from build123d import *

# Parameters (mm, degrees)
SKETCH_1_R           = 2.5
SKETCH_1_R_2         = 8
EXTRUDE_1_DEPTH      = 2
SKETCH_2_R           = 34
CUT_EXTRUDE_1_DEPTH  = 0.5
SKETCH_3_R           = 2
CUT_EXTRUDE_2_DEPTH  = 28.5
SKETCH_5_R           = 2.1
CUT_EXTRUDE_3_DEPTH  = 10
SKETCH_4_R           = 2.6
CUT_EXTRUDE_4_DEPTH  = 10
SKETCH_7_W           = 125
SKETCH_7_H           = 125
SKETCH_7_W_2         = 80
SKETCH_7_H_2         = 80
EXTRUDE_2_DEPTH      = 2
SKETCH_8_R           = 2.760887892
EXTRUDE_3_DEPTH      = 2
SKETCH_9_R           = 2.6
CUT_EXTRUDE_5_DEPTH  = 2
CUT_EXTRUDE_7_DEPTH  = 2
EXTRUDE_START        = -2
SKETCH_11_W          = 250
SKETCH_11_H          = 250
SKETCH_11_R          = 2.1
SKETCH_11_R_2        = 8
EXTRUDE_4_DEPTH      = 2
SKETCH_13_R          = 2.6
CUT_EXTRUDE_9_DEPTH  = 51
SKETCH_16_R          = 34
CUT_EXTRUDE_11_DEPTH = 1
SKETCH_18_W          = 250
SKETCH_18_H          = 250
SKETCH_18_W_2        = 90
SKETCH_18_H_2        = 90
CUT_EXTRUDE_12_DEPTH = 10
SKETCH_20_R          = 2.6
CUT_EXTRUDE_14_DEPTH = 10
SKETCH_21_R          = 8.1
CUT_EXTRUDE_15_DEPTH = 10
SKETCH_24_R          = 34.1
CUT_EXTRUDE_17_DEPTH = 1
EXTRUDE_START_2      = 1
SKETCH_25_R          = 34.1
SKETCH_25_R_2        = 2.1
SKETCH_25_R_3        = 8.1
EXTRUDE_5_DEPTH      = 1
CUT_EXTRUDE_20_DEPTH = 10
SKETCH_31_W          = 90
SKETCH_31_H          = 90
SKETCH_31_R          = 2.1
SKETCH_31_R_2        = 8.1
SKETCH_31_R_3        = 2.6
EXTRUDE_6_DEPTH      = 4
EXTRUDE_START_3      = -4
EXTRUDE_7_DEPTH      = 4
CUT_EXTRUDE_21_DEPTH = 10


with BuildPart() as part:
    # 草图1 → 凸台-拉伸1 (new body)
    with BuildSketch(Plane.XY):
        Polygon((-33, 40), (-40, 40), (-40, 33), (-40, -33), (-40, -40), (40, -40), (40, 40), (33, 40), align=None)
        with Locations((-33, -33)):
            Circle(SKETCH_1_R, mode=Mode.SUBTRACT)
        with Locations((33, -30.5)):
            Circle(SKETCH_1_R, mode=Mode.SUBTRACT)
        Circle(SKETCH_1_R_2, mode=Mode.SUBTRACT)
        with Locations((-33, 33)):
            Circle(SKETCH_1_R, mode=Mode.SUBTRACT)
        with Locations((33, 33)):
            Circle(SKETCH_1_R, mode=Mode.SUBTRACT)
    extrude(amount=EXTRUDE_1_DEPTH)

    # 草图2 → 切除-拉伸1 (cut)
    with BuildSketch(Plane.XY.offset(2)):
        Circle(SKETCH_2_R)
    extrude(amount=-CUT_EXTRUDE_1_DEPTH, mode=Mode.SUBTRACT)

    # 草图3 → 切除-拉伸2 (cut)
    with BuildSketch(Plane.XY.offset(1.5)):
        with Locations((0, 30)):
            Circle(SKETCH_3_R)
        with Locations((25.980762114, -15)):
            Circle(SKETCH_3_R)
        with Locations((-25.980762114, -15)):
            Circle(SKETCH_3_R)
    extrude(amount=-CUT_EXTRUDE_2_DEPTH, mode=Mode.SUBTRACT)

    # 草图5 → 切除-拉伸3 (cut)
    with BuildSketch(Plane.XY.offset(1.5)):
        with Locations((25.980762114, -15)):
            Circle(SKETCH_5_R)
        with Locations((0, 30)):
            Circle(SKETCH_5_R)
        with Locations((-25.980762114, -15)):
            Circle(SKETCH_5_R)
    extrude(amount=-CUT_EXTRUDE_3_DEPTH, mode=Mode.SUBTRACT)

    # 草图4 → 切除-拉伸4 (cut)
    with BuildSketch(Plane.XY.offset(2)):
        with Locations((-33, 33)):
            Circle(SKETCH_4_R)
        with Locations((33, 33)):
            Circle(SKETCH_4_R)
        with Locations((33, -30.5)):
            Circle(SKETCH_4_R)
        with Locations((-33, -33)):
            Circle(SKETCH_4_R)
    extrude(amount=-CUT_EXTRUDE_4_DEPTH, mode=Mode.SUBTRACT)

    # 草图7 → 凸台-拉伸2 (add)
    with BuildSketch(Plane(origin=(0, 0, 0), x_dir=(-1, 0, 0), z_dir=(0, 0, -1))):
        Rectangle(SKETCH_7_W, SKETCH_7_H)
        Rectangle(SKETCH_7_W_2, SKETCH_7_H_2, mode=Mode.SUBTRACT)
    extrude(amount=-EXTRUDE_2_DEPTH)

    # 草图8 → 凸台-拉伸3 (add)
    with BuildSketch(Plane(origin=(0, 0, 0), x_dir=(-1, 0, 0), z_dir=(0, 0, -1))):
        with Locations((-33, -30.5)):
            Circle(SKETCH_8_R)
    extrude(amount=-EXTRUDE_3_DEPTH)

    # 草图9 → 切除-拉伸5 (cut)
    with BuildSketch(Plane(origin=(0, 0, 0), x_dir=(-1, 0, 0), z_dir=(0, 0, -1))):
        with Locations((-33, -34.063377391)):
            Circle(SKETCH_9_R)
    extrude(amount=-CUT_EXTRUDE_5_DEPTH, mode=Mode.SUBTRACT)

    # 草图10 → 切除-拉伸7 (cut)
    with BuildSketch(Plane(origin=(0, 0, 0), x_dir=(-1, 0, 0), z_dir=(0, 0, -1))):
        with BuildLine():
            Line((13.58008401, -47.982963501), (-13.58008401, -47.982963501))
            ThreePointArc((-13.58008401, -47.982963501), (-20.483293381, -41.079754129), (-13.58008401, -34.176544757))
            Line((-13.58008401, -34.176544757), (13.58008401, -34.176544757))
            ThreePointArc((13.58008401, -34.176544757), (20.483293381, -41.079754129), (13.58008401, -47.982963501))
        make_face()
    extrude(amount=-CUT_EXTRUDE_7_DEPTH, mode=Mode.SUBTRACT)

    # 草图11 → 凸台-拉伸4 (add)
    with BuildSketch(Plane(origin=(0, 0, 0), x_dir=(-1, 0, 0), z_dir=(0, 0, -1)).offset(EXTRUDE_START)):
        Rectangle(SKETCH_11_W, SKETCH_11_H)
        with Locations(Location((25.980762114, -15, 0), (0, 0, 180))):
            Circle(SKETCH_11_R, mode=Mode.SUBTRACT)
        Circle(SKETCH_11_R_2, mode=Mode.SUBTRACT)
        with Locations(Location((-25.980762114, -15, 0), (0, 0, 180))):
            Circle(SKETCH_11_R, mode=Mode.SUBTRACT)
        with Locations(Location((0, 30, 0), (0, 0, 180))):
            Circle(SKETCH_11_R, mode=Mode.SUBTRACT)
    extrude(amount=EXTRUDE_4_DEPTH)

    # 草图13 → 切除-拉伸9 (cut)
    with BuildSketch(Plane(origin=(0, 0, 0), x_dir=(-1, 0, 0), z_dir=(0, 0, -1))):
        with Locations((-105, 105)):
            Circle(SKETCH_13_R)
        with Locations((105, 105)):
            Circle(SKETCH_13_R)
        with Locations((-105, -105)):
            Circle(SKETCH_13_R)
        with Locations((105, -98.771678495)):
            Circle(SKETCH_13_R)
    extrude(amount=-CUT_EXTRUDE_9_DEPTH, mode=Mode.SUBTRACT)

    # 草图16 → 切除-拉伸11 (cut)
    with BuildSketch(Plane.XY.offset(2)):
        Circle(SKETCH_16_R)
    extrude(amount=-CUT_EXTRUDE_11_DEPTH, mode=Mode.SUBTRACT)

    # 草图18 → 切除-拉伸12 (cut)
    with BuildSketch(Plane(origin=(0, 0, 0), x_dir=(-1, 0, 0), z_dir=(0, 0, -1))):
        Rectangle(SKETCH_18_W, SKETCH_18_H)
        Rectangle(SKETCH_18_W_2, SKETCH_18_H_2, mode=Mode.SUBTRACT)
    extrude(amount=-CUT_EXTRUDE_12_DEPTH, mode=Mode.SUBTRACT)

    # 草图20 → 切除-拉伸14 (cut)
    with BuildSketch(Plane(origin=(0, 0, 0), x_dir=(-1, 0, 0), z_dir=(0, 0, -1))):
        with Locations((-35, 35)):
            Circle(SKETCH_20_R)
        with Locations((35, 35)):
            Circle(SKETCH_20_R)
        with Locations((35, -35)):
            Circle(SKETCH_20_R)
        with Locations((-35, -35)):
            Circle(SKETCH_20_R)
    extrude(amount=-CUT_EXTRUDE_14_DEPTH, mode=Mode.SUBTRACT)

    # 草图21 → 切除-拉伸15 (cut)
    with BuildSketch(Plane.XY.offset(1)):
        Circle(SKETCH_21_R)
    extrude(amount=-CUT_EXTRUDE_15_DEPTH, mode=Mode.SUBTRACT)

    # 草图24 → 切除-拉伸17 (cut)
    with BuildSketch(Plane.XY.offset(2)):
        Circle(SKETCH_24_R)
    extrude(amount=-CUT_EXTRUDE_17_DEPTH, mode=Mode.SUBTRACT)

    # 草图25 → 凸台-拉伸5 (add)
    with BuildSketch(Plane.XY.offset(1).offset(EXTRUDE_START_2)):
        Circle(SKETCH_25_R)
        with Locations((25.980762114, -15)):
            Circle(SKETCH_25_R_2, mode=Mode.SUBTRACT)
        with Locations((0, 30)):
            Circle(SKETCH_25_R_2, mode=Mode.SUBTRACT)
        Circle(SKETCH_25_R_3, mode=Mode.SUBTRACT)
        with Locations((-25.980762114, -15)):
            Circle(SKETCH_25_R_2, mode=Mode.SUBTRACT)
    extrude(amount=-EXTRUDE_5_DEPTH)

    # 草图30 → 切除-拉伸20 (cut)
    with BuildSketch(Plane(origin=(0, 0, 0), x_dir=(-1, 0, 0), z_dir=(0, 0, -1))):
        with BuildLine():
            Line((-34.25879914, 10.195171229), (-25.460402767, 24.557274857))
            ThreePointArc((-25.460402767, 24.557274857), (-19.205340885, 26.059890654), (-17.702725087, 19.804828771))
            Line((-17.702725087, 19.804828771), (-26.50112146, 5.442725143))
            ThreePointArc((-26.50112146, 5.442725143), (-32.756183343, 3.940109346), (-34.25879914, 10.195171229))
        make_face()
    extrude(amount=-CUT_EXTRUDE_20_DEPTH, mode=Mode.SUBTRACT)

    # 草图31 → 凸台-拉伸6 (add)
    with BuildSketch(Plane.XY):
        Rectangle(SKETCH_31_W, SKETCH_31_H)
        with Locations((-25.980762114, -15)):
            Circle(SKETCH_31_R, mode=Mode.SUBTRACT)
        Circle(SKETCH_31_R_2, mode=Mode.SUBTRACT)
        with Locations((0, 30)):
            Circle(SKETCH_31_R, mode=Mode.SUBTRACT)
        with Locations((25.980762114, -15)):
            Circle(SKETCH_31_R, mode=Mode.SUBTRACT)
        with Locations(Location((-35, 35, 0), (0, 0, 180))):
            Circle(SKETCH_31_R_3, mode=Mode.SUBTRACT)
        with Locations(Location((35, 35, 0), (0, 0, 180))):
            Circle(SKETCH_31_R_3, mode=Mode.SUBTRACT)
        with Locations(Location((-35, -35, 0), (0, 0, 180))):
            Circle(SKETCH_31_R_3, mode=Mode.SUBTRACT)
        with Locations(Location((35, -35, 0), (0, 0, 180))):
            Circle(SKETCH_31_R_3, mode=Mode.SUBTRACT)
        with BuildLine():
            Line((17.702725087, 19.804828771), (26.50112146, 5.442725143))
            ThreePointArc((26.50112146, 5.442725143), (32.756183343, 3.940109346), (34.25879914, 10.195171229))
            Line((34.25879914, 10.195171229), (25.460402767, 24.557274857))
            ThreePointArc((25.460402767, 24.557274857), (19.205340885, 26.059890654), (17.702725087, 19.804828771))
        make_face(mode=Mode.SUBTRACT)
    extrude(amount=EXTRUDE_6_DEPTH)

    # 草图32 → 凸台-拉伸7 (add)
    with BuildSketch(Plane.XY.offset(4).offset(EXTRUDE_START_3)):
        with BuildLine():
            Line((17.702725087, 19.804828771), (26.50112146, 5.442725143))
            ThreePointArc((26.50112146, 5.442725143), (32.756183343, 3.940109346), (34.25879914, 10.195171229))
            Line((34.25879914, 10.195171229), (25.460402767, 24.557274857))
            ThreePointArc((25.460402767, 24.557274857), (19.205340885, 26.059890654), (17.702725087, 19.804828771))
        make_face()
    extrude(amount=EXTRUDE_7_DEPTH)

    # 草图33 → 切除-拉伸21 (cut)
    with BuildSketch(Plane(origin=(0, 0, 0), x_dir=(-1, 0, 0), z_dir=(0, 0, -1))):
        with BuildLine():
            Line((31.466175781, 0.279206161), (19.18721424, 24.940909849))
            ThreePointArc((19.18721424, 24.940909849), (21.75266604, 32.594262797), (29.406018987, 30.028810997))
            Line((29.406018987, 30.028810997), (41.684980529, 5.367107309))
            ThreePointArc((41.684980529, 5.367107309), (39.119528729, -2.286245639), (31.466175781, 0.279206161))
        make_face()
    extrude(amount=-CUT_EXTRUDE_21_DEPTH, mode=Mode.SUBTRACT)


solid = part.part
For this review, take the finished solid that the model builds, in its own axes (mm). A direction names the side the tool comes from. Coordinates: 2 decimals unless noted, no trailing zeros. Order: outer loops, then holes, each group sorted by start corner. A loop starts at its lowest first (then second) coordinate and runs counter-clockwise, first axis right, second up. Notation, with made-up numbers: (30.25, -12) - (41.25, -12) arc R21 cw to (41.25, -3) - close; hole circle Ø1 at (-18, 47.5). An arc over 180 degrees is marked (long way). Use one line per item in the form item = value.
Q1. Consider section A-A (y = -35). Give the boundary of the cut face in (x, z), then the cut area to 3 significant figures.
Checked values:
outline = (-45, 0) - (-37.6, 0) - (-37.6, 4) - (-45, 4) - close; (-32.4, 0) - (32.4, 0) - (32.4, 4) - (-32.4, 4) - close; (37.6, 0) - (45, 0) - (45, 4) - (37.6, 4) - close
area = 318 mm2
Q2. Consider section C-C (z = 2.45). Give the number of separate pieces and of enclosed holes in the cut face, then the cut area to 3 significant figures.
Checked values:
separate_pieces = 1
enclosed_holes = 9
area = 7,350 mm2
Q3. Consider section D-D (x = -35). Give the boundary of the cut face in (y, z).
Checked values:
outline = (-45, 0) - (-37.6, 0) - (-37.6, 4) - (-45, 4) - close; (-32.4, 0) - (-2.66, 0) - (-2.66, 4) - (-32.4, 4) - close; (18.79, 0) - (32.4, 0) - (32.4, 4) - (18.79, 4) - close; (37.6, 0) - (45, 0) - (45, 4) - (37.6, 4) - close
Q4. For P1, Ø6, axis at x = 35, y = 35, coming from the +Z side; P2, Ø3.5, axis at x = -25.98, y = -15, coming from the +Z side, all flat-tipped, find the tip position at first contact; note any pin that passes through.
Checked values:
P1 = 4
P2 = through
Q5. Draft analysis for pull direction Y (two halves, no side actions). For faces 3 (the flat face through (9, 1, 0)), 4 (the cylindrical face through (-0.46, 27.95, 2.03)), 5 (the flat face through (1, -45, 2)), state which applies: +Y half, -Y half, draft (parallel to the pull), parting line (faces both ways), or undercut.
Checked values:
face_3 = draft
face_4 = undercut
face_5 = -Y half
Q6. Consider section B-B (x = 0). Give the boundary of the cut face in (y, z).
Checked values:
outline = (-45, 0) - (-8.1, 0) - (-8.1, 4) - (-45, 4) - close; (8.1, 0) - (27.9, 0) - (27.9, 4) - (8.1, 4) - close; (32.1, 0) - (45, 0) - (45, 4) - (32.1, 4) - close
Q7. For probe 1 along X at (y, z) = (35, 2.65); probe 2 along Y at (x, z) = (0, 1.35), list the stretches that pass through material, from the lowest coordinate up. Write a range as from..to.
Checked values:
probe_1 = -45..-37.6, -32.4..32.4, 37.6..45
probe_2 = -45..-8.1, 8.1..27.9, 32.1..45
Q8. For faces 1 (the flat face through (9, 1, 4)), 2 (the flat face through (-35.46, 17.87, 1.97)), list the 3-axis set-ups (+Z, -Z, +X, -X, +Y, -Y) from which the entire face can be reached by the end or side of a thin tool; tool diameter is ignored.
Checked values:
face_1 = +Z, +X, -X, +Y, -Y
face_2 = +Z, -Z
